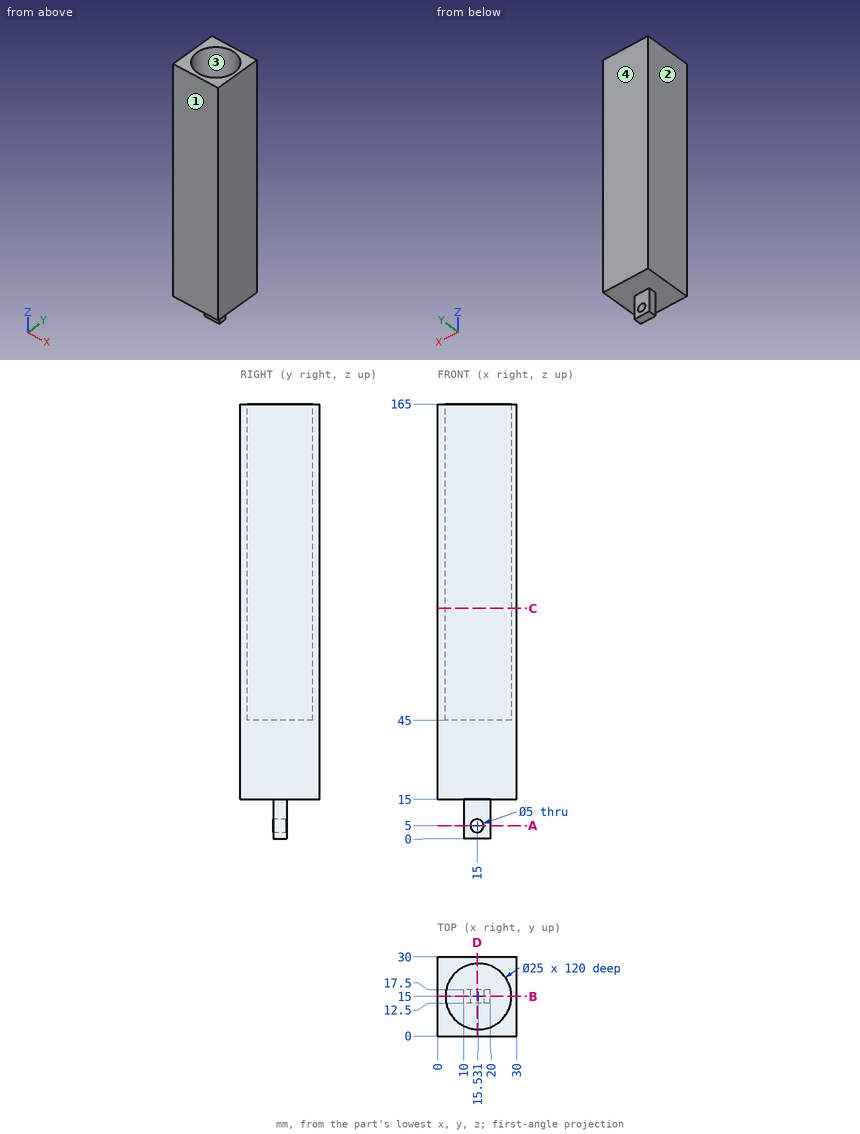
Check sheet for the drawn part. Datum: minimum x, y, z corner. Units: mm. Coordinates: 2 decimals unless noted, no trailing zeros. Order: outer loops, then holes, each group sorted by start corner. A loop starts at its lowest first (then second) coordinate and runs counter-clockwise, first axis right, second up. Notation, with made-up numbers: M 48.5,-20 L 95.5,-20 A15 cw 95.5,-10 Z; hole C 17,22 d3. An arc over 180 degrees is marked long. One line per item, written item: value. Start each with the question number.
Item 1: Sectioned sample at C-C (z = 87.5). Enter the section's corners in (x, y).
Item 2: Mould release check, pull along Y, two halves, no side actions. Record for the marked faces 1, 2, 3 and 4: released by +Y, released by -Y, zero draft, split by the parting line, or undercut.
Item 3: Sectioned sample at D-D (x = 15). Enter the section's corners in (y, z).
Item 4: Sectioned sample at A-A (z = 5). Enter the section's corners in (x, y).
Item 5: Sectioned sample at B-B (y = 15). Enter the section's corners in (x, z).
Item 6: Gauge pin test, flat ends, axial feed: pin 1 (5 mm diameter, centred on x = 7, y = 18, fed in from -Z); pin 2 (5 mm diameter, centred on x = 15, z = 9, fed in from +Y); pin 3 (8 mm diameter, centred on y = 17.5, z = 108.5, fed in from -X); pin 4 (5.5 mm diameter, centred on y = 14.5, z = 4.5, fed in from +X). Record the tip position at first contact, or that the pin passes through.
Item 7: Scan lines: probe 1 along Y at (x, z) = (15.75, 121); probe 2 along X at (y, z) = (16.1, 5); probe 3 along Z at (x, y) = (11.5, 14). Record each from-to range of solid material in increasing order.
Conclusion:
1. outline: M 0,0 L 30,0 L 30,30 L 0,30 Z; hole C 15.53,15 d25
2. face 1: released by -Y
2. face 2: zero draft
2. face 3: undercut
2. face 4: released by +Y
3. outline: M 0,15 L 12.5,15 L 12.5,7.5 L 17.5,7.5 L 17.5,15 L 30,15 L 30,165 L 27.49,165 L 27.49,45 L 2.51,45 L 2.51,165 L 0,165 Z; M 12.5,0 L 17.5,0 L 17.5,2.5 L 12.5,2.5 Z
4. outline: M 10,12.5 L 12.5,12.5 L 12.5,17.5 L 10,17.5 Z; M 17.5,12.5 L 20,12.5 L 20,17.5 L 17.5,17.5 Z
5. outline: M 0,15 L 10,15 L 10,0 L 20,0 L 20,15 L 30,15 L 30,165 L 28.03,165 L 28.03,45 L 3.03,45 L 3.03,165 L 0,165 Z; hole C 15,5 d5
6. pin 1: stops at z = 15
6. pin 2: stops at y = 17.5
6. pin 3: stops at x = 0
6. pin 4: stops at x = 20
7. probe 1: y = 0 to 2.5, 27.5 to 30
7. probe 2: x = 10 to 12.5, 17.5 to 20
7. probe 3: z = 0 to 45
